from build123d import *
from build123d.topology import SkipClean

# Parameters (mm, degrees)
SKETCH_1_R          = 17
EXTRUDE_1_DEPTH     = 4
SKETCH_2_R          = 2
CUT_EXTRUDE_1_DEPTH = 3
SKETCH_2_3_R        = 2
EXTRUDE_2_DEPTH     = 2
CUT_EXTRUDE_START   = -3
CUT_EXTRUDE_2_DEPTH = 3


with BuildPart() as part:
    # Sketch 1 → Extrude 1 (new body)
    with BuildSketch(Plane(origin=(0, 0, 0), x_dir=(1, 0, 0), z_dir=(0, 1, 0))):
        with Locations(Location((0, 0, 0), (0, 0, 270))):
            Circle(SKETCH_1_R)
    extrude(amount=EXTRUDE_1_DEPTH)

    # Sketch 2 → Cut-Extrude 1 (cut)
    with BuildSketch(Plane(origin=(0, 4, 0), x_dir=(1, 0, 0), z_dir=(0, 1, 0))):
        with Locations(Location((-7.778174593, 7.778174593, 0), (0, 0, 270))):
            Circle(SKETCH_2_R)
        with Locations(Location((7.778174593, 7.778174593, 0), (0, 0, 270))):
            Circle(SKETCH_2_R)
    extrude(amount=-CUT_EXTRUDE_1_DEPTH, mode=Mode.SUBTRACT)

    # Sketch 2_3 → Extrude 2 (add)
    with BuildSketch(Plane(origin=(0, 4, 0), x_dir=(1, 0, 0), z_dir=(0, 1, 0))):
        with Locations(Location((11, 0, 0), (0, 0, 270))):
            Circle(SKETCH_2_3_R)
        with Locations(Location((-11, 0, 0), (0, 0, 270))):
            Circle(SKETCH_2_3_R)
    extrude(amount=EXTRUDE_2_DEPTH)

    # Sketch 4 → Cut-Extrude 2 (cut)
    with SkipClean():  # the faces are left unmerged after this step: merging them gives an invalid solid
        with BuildSketch(Plane.XZ.offset(CUT_EXTRUDE_START)):
            with BuildLine():
                ThreePointArc((-9.192388155, -9.192388155), (0, -13), (9.192388155, -9.192388155))
                ThreePointArc((9.192388155, -9.192388155), (9.192388155, -6.363961031), (6.363961031, -6.363961031))
                ThreePointArc((6.363961031, -6.363961031), (0, -9), (-6.363961031, -6.363961031))
                ThreePointArc((-6.363961031, -6.363961031), (-9.192388155, -6.363961031), (-9.192388155, -9.192388155))
            make_face()
            with BuildLine():
                ThreePointArc((-9.192388155, 9.192388155), (0, 13), (9.192388155, 9.192388155))
                ThreePointArc((9.192388155, 9.192388155), (9.192388155, 6.363961031), (6.363961031, 6.363961031))
                ThreePointArc((6.363961031, 6.363961031), (0, 9), (-6.363961031, 6.363961031))
                ThreePointArc((-6.363961031, 6.363961031), (-9.192388155, 6.363961031), (-9.192388155, 9.192388155))
            make_face()
        extrude(amount=CUT_EXTRUDE_2_DEPTH, mode=Mode.SUBTRACT)


solid = part.part
Here's how the part is built. I have some questions about the finished solid (model axes, mm). A direction names the side the tool comes from. Round coordinates to 2 decimals unless told otherwise and drop trailing zeros. Order: outer loops, then holes, each group sorted by start corner. A loop starts at its lowest first (then second) coordinate and runs counter-clockwise, first axis right, second up. Notation, with made-up numbers: M 3.25,-33 L 34.25,-33 A27 cw 34.25,-3 Z; hole C 56,-14 d11. An arc over 180 degrees is marked long. Return JSON: item names as keys, results as strings. Group by question number.
1. I'm going to push flat-ended pins straight in: pin 1 Ø2 at (x, z) = (2.5, -11) entering from -Y; pin 2 Ø10 at (x, z) = (10.5, -6.5) entering from +Y; pin 3 Ø6.5 at (x, z) = (-7.78, -7.78) entering from +Y; pin 4 Ø3.5 at (x, z) = (7.78, -7.78) entering from -Y. Where does each tip first touch, or does it pass through?
2. On a 3-axis mill with a long thin cutter (end or side, diameter ignored), from which of +Z, -Z, +X, -X, +Y, -Y can I reach the whole of each face in a straight line? I mean faces 1 (the face through (0, 3, -10)), 2 (the face through (-9, 5, 0)), 3 (the face through (11, 6, 0)). Say none if no direction works.
3. If we section it at C-C on z = 0: List the corners of the cut face in (x, y) for me.
4. If we section it at D-D on y = 5.55: List the corners of the cut face in (x, z) for me, then the cut area to 3 significant figures.
5. If we section it at B-B on x = 0: List the corners of the cut face in (y, z) for me, then the cut area to 3 significant figures.
6. If we mould it in two halves opening along X, with no side actions, what happens to faces 4 (the face through (0, 0, 0)), 5 (the face through (-9.16, 1.52, 6.33)), 6 (the face through (16.855, 1.972, -2.213))? For each: pulls with the +X half, pulls with the -X half, needs draft (parallel to the pull), parting line crosses it, or undercut.
7. If we section it at A-A on y = 2.45: List the corners of the cut face in (x, z) for me.
8. Please list where these lines run through material, in increasing order: probe 1 along Z at (x, y) = (9, 0.4); probe 2 along Z at (x, y) = (-4.5, 2.95); probe 3 along X at (y, z) = (5, 0).
Reply:
{
 "1": {"pin 1": "y = 3", "pin 2": "y = 6", "pin 3": "y = 4", "pin 4": "through"},
 "2": {"face 1": "-Y", "face 2": "+Y", "face 3": "+Z, -Z, +X, -X, +Y"},
 "3": {"outline": "M -17,0 L 17,0 L 17,4 L 13,4 L 13,6 L 9,6 L 9,4 L -9,4 L -9,6 L -13,6 L -13,4 L -17,4 Z"},
 "4": {"outline": "C -11,0 d4; C 11,0 d4", "area": "25.1 mm^2"},
 "5": {"outline": "M 0,-17 L 4,-17 L 4,17 L 0,17 L 0,13 L 3,13 L 3,9 L 0,9 L 0,-9 L 3,-9 L 3,-13 L 0,-13 Z", "area": "112 mm^2"},
 "6": {"face 4": "needs draft", "face 5": "undercut", "face 6": "parting line crosses it"},
 "7": {"outline": "C 0,0 d34; hole M -9.19,-9.19 A13 ccw 9.19,-9.19 A2 ccw 6.36,-6.36 A9 cw -6.36,-6.36 A2 ccw Z; hole M -9.19,9.19 A2 ccw -6.36,6.36 A9 cw 6.36,6.36 A2 ccw 9.19,9.19 A13 ccw Z"},
 "8": {"probe 1": "-14.42 to -9.38, -6.19 to 6.19, 9.38 to 14.42", "probe 2": "-16.39 to -12.2, -7.79 to 7.79, 12.2 to 16.39", "probe 3": "-13 to -9, 9 to 13"}
}
